The drawing under review shows one solid part. Ordinate dimensions are in mm from its lowest x, y, z. Give positions to 0.01 mm unless a question says otherwise; leave off trailing zeros. Loops run counter-clockwise (first coordinate to the right, second up) from the corner with the lowest first, then second, coordinate; pieces in that order, holes last. Notation, with made-up numbers: M 11.5,-27 L 53.5,-27 A20 ccw 53.5,-7 Z; hole C 61.5,42.5 d9. An arc over 180 degrees is marked long. Write item = value, one per line. Start each with the question number.
1. We need section A-A on z = 4.55. Give the boundary of the cut face in (x, y), then the cut area to 3 significant figures.
2. We need section C-C on x = 29. Give the boundary of the cut face in (y, z).
3. We need section B-B on y = 152. Give the boundary of the cut face in (x, z), then the cut area to 3 significant figures.
4. For pin 1 (3 mm diameter, centred on y = 82, z = 2, fed in from -X), flat-tipped, find the tip position at first contact; note if it passes through.
5. Wall thickness on line 1 along X through (y, z) = (54, 1.3) (1 decimal); line 2 along X through (y, z) = (29.5, 0.8): over which ranges is each line inside the solid? List them lowest first. Write a range as from..to.
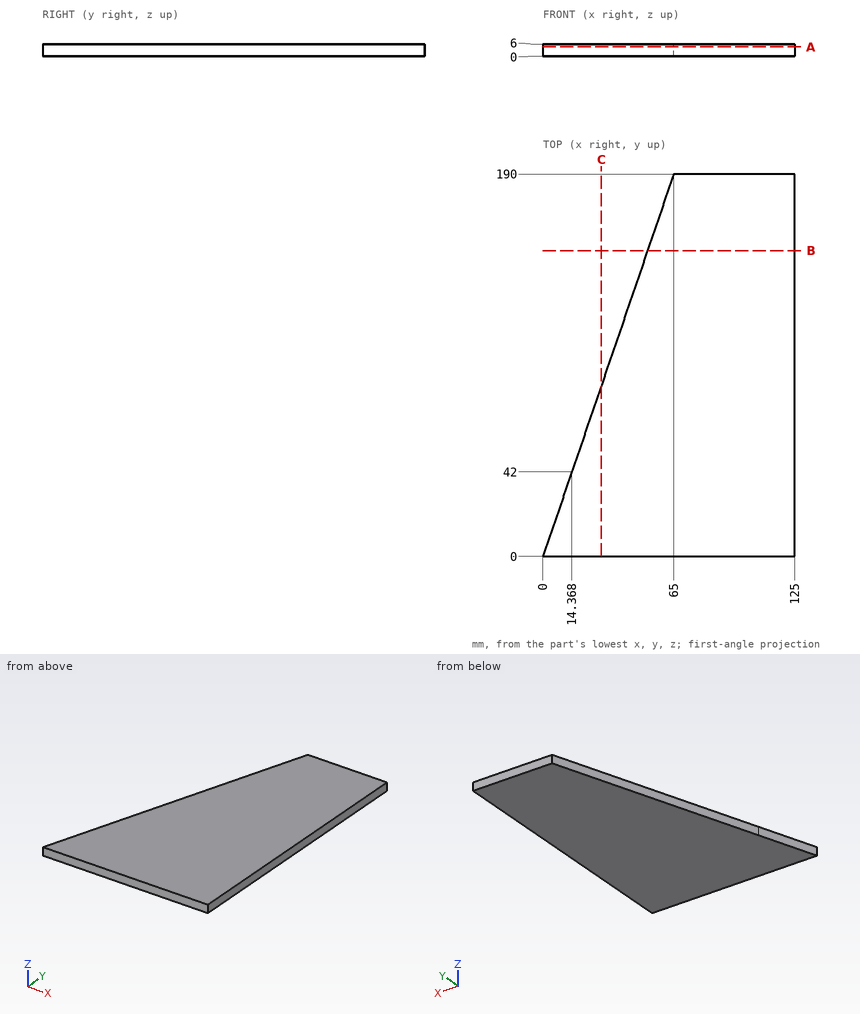
Final values:
q1.outline = M 0,0 L 125,0 L 125,190 L 65,190 Z
q1.area = 17,600 mm²
q2.outline = M 0,0 L 84.77,0 L 84.77,6 L 0,6 Z
q3.outline = M 52,0 L 125,0 L 125,6 L 52,6 Z
q3.area = 438 mm²
q4.pin_1 = 27.54
q5.line_1 = 18.5..125
q5.line_2 = 10.09..125
